from build123d import *

# Parameters (mm, degrees)
F0_W     = 200
F0_H     = 150
F1_DEPTH = 4
F3_DEPTH = 25


with BuildPart() as f1:
    # F0 (on Top) → F1 (new body)
    with BuildSketch(Plane.XY):
        Rectangle(F0_W, F0_H)
    extrude(amount=F1_DEPTH)

    # F2 (on face) → F3 (cut)
    with BuildSketch(Plane.XY.offset(4)):
        Polygon((-87.500563, 60.43724), (87.499437, 60.43724), (87.499437, -64.56276), (-77.500563, -64.56276), (-87.500563, -64.56276), (-87.500563, -38.276056), (-46.000563, -38.276056), (-41.000563, -38.276056), (-33.500563, -38.276056), (-33.500563, -30.276056), (-38.500563, -30.276056), (-38.500563, -33.276056), (-87.500563, -33.276056), (-87.500563, -6.86276), (-92.500563, -3.86276), (-100, -3.86276), (-100, -75), (100, -75), (100, 75), (-100, 75), (-100, -0.26276), (-92.500563, -0.26276), (-87.500563, 2.73724), (-87.500563, 29.723944), (-46.000563, 29.723944), (-38.500563, 29.723944), (-38.500563, 26.723944), (-33.500563, 26.723944), (-33.500563, 34.723944), (-41.000563, 34.723944), (-87.500563, 34.723944), align=None)
        with BuildLine():
            Line((60.637614, 50.43724), (-74.362386, 50.43724))
            Line((-74.362386, 50.43724), (-77.362386, 50.43724))
            Line((-77.362386, 50.43724), (-77.362386, 47.43724))
            Line((-77.362386, 47.43724), (-74.362386, 47.43724))
            Line((-74.362386, 47.43724), (57.637614, 47.43724))
            Line((57.637614, 47.43724), (60.637614, 47.43724))
            Line((60.637614, 47.43724), (69.499437, 47.43724))
            ThreePointArc((69.499437, 47.43724), (73.034971, 45.972774), (74.499437, 42.43724))
            Line((74.499437, 42.43724), (74.499437, -46.56276))
            ThreePointArc((74.499437, -46.56276), (73.034971, -50.098294), (69.499437, -51.56276))
            Line((69.499437, -51.56276), (60.637614, -51.56276))
            Line((60.637614, -51.56276), (-77.500563, -51.56276))
            Line((-77.500563, -51.56276), (-77.500563, -54.56276))
            Line((-77.500563, -54.56276), (60.637614, -54.56276))
            Line((60.637614, -54.56276), (77.499437, -54.56276))
            Line((77.499437, -54.56276), (77.499437, 47.43724))
            Line((77.499437, 47.43724), (77.499437, 50.43724))
            Line((77.499437, 50.43724), (74.499437, 50.43724))
            Line((74.499437, 50.43724), (60.637614, 50.43724))
        make_face()
    extrude(amount=-F3_DEPTH, mode=Mode.SUBTRACT)


solid = f1.part
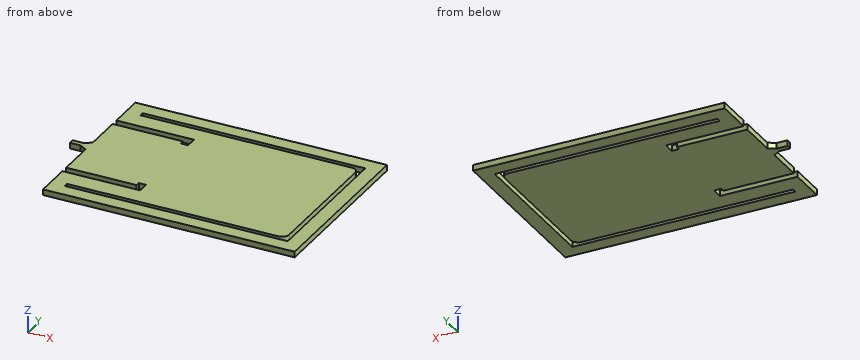
Build history of the part. All positions in model axes, mm. Give positions to 0.01 mm unless a question says otherwise; leave off trailing zeros. Loops run counter-clockwise (first coordinate to the right, second up) from the corner with the lowest first, then second, coordinate; pieces in that order, holes last. Notation, with made-up numbers: (66.25, 65.5) - (103.25, 65.5) arc R23 ccw to (103.25, 84.5) - close; hole circle Ø11 at (41, 24). An arc over 180 degrees is marked (long way). Write item = value, one per line. Start each with the question number.
1) Probe probe 1 along Y at (x, z) = (-2.5, 2.6); probe 2 along Y at (x, z) = (-68.5, 3.4); probe 3 along X at (y, z) = (-39, 0.6). List the from-to ranges inside material, lowest first. Write a range as from..to.
2) Drop a flat-ended pin along its axis: pin 1 Ø1.2 at (y, z) = (-33, 1.5) entering from -X. Give the stop position or say it passes through.
3) Band-saw the part on B-B on y = 5. Give the cut face in (x, z).
4) Band-saw the part on D-D on x = 64.5. Give the cut face in (y, z), plus the area to 3 significant figures.
5) Band-saw the part on A-A on x = -83. Give the cut face in (y, z).
Final values:
q1.probe_1 = -64.56..-54.56, -51.56..47.44, 50.44..60.44
q1.probe_2 = -64.56..-54.56, -51.56..-38.28, -33.28..29.72, 34.72..47.44, 50.44..60.44
q1.probe_3 = -87.5..74.5, 77.5..87.5
q2.pin_1 = -87.5
q3.outline = (-87.5, 0) - (74.5, 0) - (74.5, 4) - (-87.5, 4) - close; (77.5, 0) - (87.5, 0) - (87.5, 4) - (77.5, 4) - close
q4.outline = (-64.56, 0) - (-54.56, 0) - (-54.56, 4) - (-64.56, 4) - close; (-51.56, 0) - (47.44, 0) - (47.44, 4) - (-51.56, 4) - close; (50.44, 0) - (60.44, 0) - (60.44, 4) - (50.44, 4) - close
q4.area = 476 mm²
q5.outline = (-64.56, 0) - (-38.28, 0) - (-38.28, 4) - (-64.56, 4) - close; (-33.28, 0) - (29.72, 0) - (29.72, 4) - (-33.28, 4) - close; (34.72, 0) - (60.44, 0) - (60.44, 4) - (34.72, 4) - close
